Autodesk Inventor part; units mm, degrees
ref_plane "YZ Plane" through (0, 0, 0) normal (1, 0, 0) x (0, 1, 0)
ref_plane "XZ Plane" through (0, 0, 0) normal (0, 1, 0) x (-1, 0, 0)
ref_plane "XY Plane" through (0, 0, 0) normal (0, 0, 1) x (1, 0, 0)
sketch "Skizze1" plane through (0, 0, 0) normal (0, 0, 1) x (1, 0, 0)
  line L0 (-28.13, 28.13) -> (28.13, 28.13)
  line L1 (28.13, 28.13) -> (28.13, -28.13)
  line L2 (28.13, -28.13) -> (-28.13, -28.13)
  line L3 (-28.13, -28.13) -> (-28.13, 28.13)
  line L4 (-39.382, 0) -> (39.382, 0) construction
  line L5 (0, -39.382) -> (0, 39.382) construction
  point P0 (0, 0)
  dimension "d0" = 56.26
extrude "Extrusion1" add sketch "Skizze1" along normal blind 1.6
sketch "Skizze2" plane through (0, 0, 1.6) normal (0, 0, 1) x (1, 0, 0)
  line L0 (0, -39.382) -> (0, 39.382) construction
  line L1 (-39.382, 0) -> (39.382, 0) construction
  line L2 (-26.6175, 26.6175) -> (26.6175, 26.6175)
  line L3 (26.6175, 26.6175) -> (26.6175, -26.6175)
  line L4 (26.6175, -26.6175) -> (-26.6175, -26.6175)
  line L5 (-26.6175, -26.6175) -> (-26.6175, 26.6175)
  line L6 (28.13, 28.13) -> (-28.13, 28.13)
  point P0 (0, 0)
  dimension "d3" = 53.235
extrude "Extrusion2" add sketch "Skizze2" along normal blind 2.5
sketch "Skizze3" plane through (0, 0, 0) normal (0, 0, -1) x (-1, 0, 0)
  line L0 (28.13, -28.13) -> (-28.13, -28.13)
  line L1 (28.13, 28.13) -> (28.13, -28.13)
  line L2 (-28.13, 28.13) -> (28.13, 28.13)
  line L3 (-28.13, -28.13) -> (-28.13, 28.13)
  line L4 (-6.21, 20.195) -> (2.33, 20.195)
  line L5 (2.33, 20.195) -> (2.33, 7.76)
  line L6 (2.33, 7.76) -> (-6.21, 7.76)
  line L7 (-6.21, 7.76) -> (-6.21, 20.195)
  point P0 (0, 0)
  point P1 (0, 0)
  dimension "d6" = 21.92
  dimension "d7" = 8.54
  dimension "d8" = 12.435
  dimension "d9" = 35.89
extrude "Extrusion3" cut sketch "Skizze3" against normal up to surface (4.1 mm away) contours L4 L5 L6 L7
pattern_circular "Runde Anordnung1" count 4 over 360 about axis through (0, 0, -10) along (0, 0, 1) of "Extrusion3"
sketch "Skizze4" plane through (0, 0, 0) normal (0, 0, -1) x (-1, 0, 0)
  line L0 (-28.13, -28.13) -> (-28.13, 28.13)
  line L1 (-28.13, 28.13) -> (28.13, 28.13)
  point P0 (0, 0)
  point P1 (-11.817, 11.817)
  dimension "d15" = 16.313
  dimension "d16" = 16.313
hole "Bohrung1" at (11.817, 11.817, 0) direction (0, 0, 1) diameter 5.333 depth 3.35 counterbore diameter 8.2 counterbore depth 2.2
pattern_circular "Runde Anordnung2" count 4 over 360 about axis through (0, 0, -10) along (0, 0, 1) of "Bohrung1"
sketch "Skizze5" plane through (0, 0, 0) normal (0, 0, -1) x (-1, 0, 0)
  point P0 (0, 0)
  point P1 (0, 0)
hole "Bohrung2" at (0, 0, 0) direction (0, 0, 1) diameter 5.333 depth 3.35 counterbore diameter 11.199 counterbore depth 2.2
properties part number "PCB_cover_platte_0,1_reduziert"
Part model, mm, in its own coordinate system. A direction names the side the tool comes from. Coordinates: 2 decimals unless noted, no trailing zeros. Loops run counter-clockwise (first coordinate to the right, second up) from the corner with the lowest first, then second, coordinate; pieces in that order, holes last. Notation, with made-up numbers: (85.5, -7.5) -> (143.5, -7.5) arc R15 ccw to (143.5, 8.5) -> close; hole circle Ø7 at (7, 16.25). An arc over 180 degrees is marked (long way). Use a Markdown table: item, result. Add a question column.
Item 1: Band-saw the part on A-A on y = 0. Give the number of separate pieces and of enclosed holes in the cut face, plus the area to 3 significant figures.
Item 2: Band-saw the part on D-D on y = 18. Write the cut outline in (x, z), plus the area to 3 significant figures.
Item 3: Band-saw the part on B-B on x = 18.5. Write the cut outline in (y, z).
Item 4: Which spindle directions (+Z, -Z, +X, -X, +Y, -Y) get a long thin tool onto all of the face, cutting with end or side? Do faces 5 (the flat face through (-12, 12, 3.35)), 6 (the flat face through (2, 7.76, 2)), 7 (the flat face through (0, 26.618, 3)). Say none if no direction does.
Item 5: Pull direction Y, two halves, no side cores. Call faces 1 (the flat face through (-6.21, -14, 2)), 2 (the flat face through (0, -28.13, 1)), 3 (the flat face through (28.13, 0, 1)), 4 (the flat face through (12.7, -14.5, 2.2)): +Y half, -Y half, draft (parallel to the pull), parting line (faces both ways), or undercut.
Item 6: Flat gauge pins, fed straight in: P1, Ø2, axis at y = 14, z = 3, coming from the -X side; P2, Ø4.5, axis at x = -11.817, y = -11.817, coming from the -Z side; P3, Ø4.5, axis at x = -11.5, y = -12.5, coming from the -Z side. Where does each tip first touch, or does it go through?
Item 7: Probe probe 1 along X at (y, z) = (0, 2.85) (1 decimal); probe 2 along X at (y, z) = (1, 2.4) (1 decimal); probe 3 along Y at (x, z) = (10, 3.2). List the from-to ranges inside material, lowest first.
Geometry says:
| question | item | result |
|---|---|---|
| 1 | separate pieces | 3 |
| 1 | enclosed holes | 0 |
| 1 | area | 90.4 mm² |
| 2 | outline | (-28.13, 0) -> (-2.33, 0) -> (-2.33, 4.1) -> (-26.62, 4.1) -> (-26.62, 1.6) -> (-28.13, 1.6) -> close; (6.21, 0) -> (28.13, 0) -> (28.13, 1.6) -> (26.62, 1.6) -> (26.62, 4.1) -> (6.21, 4.1) -> close |
| 2 | area | 188 mm² |
| 3 | outline | (-28.13, 0) -> (-6.21, 0) -> (-6.21, 4.1) -> (-26.62, 4.1) -> (-26.62, 1.6) -> (-28.13, 1.6) -> close; (2.33, 0) -> (28.13, 0) -> (28.13, 1.6) -> (26.62, 1.6) -> (26.62, 4.1) -> (2.33, 4.1) -> close |
| 4 | face 5 | -Z |
| 4 | face 6 | +Z, -Z |
| 4 | face 7 | +Z, +X, -X, +Y |
| 5 | face 1 | undercut |
| 5 | face 2 | -Y half |
| 5 | face 3 | draft |
| 5 | face 4 | undercut |
| 6 | P1 | x = -26.62 |
| 6 | P2 | z = 3.35 |
| 6 | P3 | z = 2.2 |
| 7 | probe 1 | -26.6 to -20.2, -7.8 to -2.7, 2.7 to 7.8, 20.2 to 26.6 |
| 7 | probe 2 | -26.6 to -20.2, -7.8 to -2.5, 2.5 to 7.8, 20.2 to 26.6 |
| 7 | probe 3 | -26.62 to -13.77, -9.87 to -6.21, 2.33 to 9.87, 13.77 to 26.62 |
